The listing builds one solid part. Answer for the finished solid, in the listing's coordinates (mm). Face numbers are marked on the shaded views. Coordinates: 2 decimals unless noted, no trailing zeros. Loops run counter-clockwise (first coordinate to the right, second up) from the corner with the lowest first, then second, coordinate; pieces in that order, holes last. Notation, with made-up numbers: (-10.75, 58.5) - (8.25, 58.5) arc R32 ccw to (8.25, 97.5) - close; hole circle Ø11 at (9, 89.25). An arc over 180 degrees is marked (long way). Return JSON: item names as keys, results as strings. Group by question number.
1. Section C-C (z = 23) is taken. Write down the section's boundary in (x, y), and give its area (3 significant figures).
2. Each of these flat-tipped pins is pushed along its axis until it touches: P1, Ø3, axis at x = -8, y = -12, coming from the +Z side; P2, Ø3, axis at x = 7.5, y = -9.5, coming from the -Z side; P3, Ø2.5, axis at x = -13, y = -13, coming from the +Z side; P4, Ø4, axis at y = -3, z = 24.5, coming from the -X side. Where does it stop, or does it pass through?
3. Section B-B (x = -13) is taken. Write down the section's boundary in (y, z), and give its area (3 significant figures).
4. Section A-A (y = 0) is taken. Write down the section's boundary in (x, z).
5. Find the intervals of material crossed by line 1 along Y through (x, z) = (13, 15.95); line 2 along Z through (x, y) = (16, 2.5); line 3 along Z through (x, y) = (0.5, 7), in increasing order.
6. Section D-D (y = 4.5) is taken. Write down the section's boundary in (x, z).
7. The mould has two halves that part along Y. Classify the marked faces 1, 2 and 3: pulls with the +Y half, pulls with the -Y half, needs draft (parallel to the pull), parting line crosses it, or undercut.
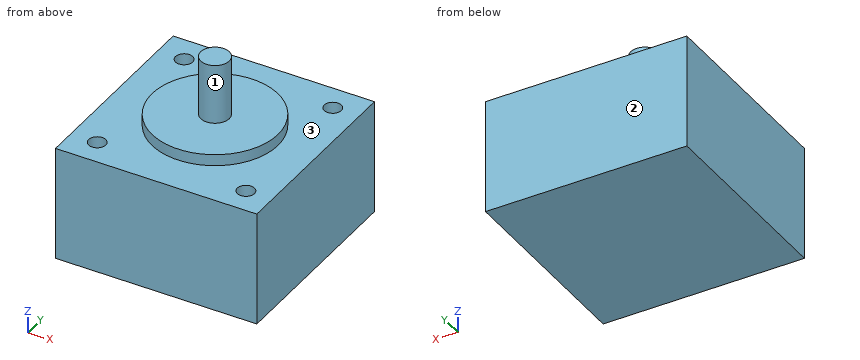
```python
from build123d import *

# Parameters (mm, degrees)
F0_W     = 35.2
F0_H     = 35.2
F1_DEPTH = 20
F2_R     = 11
F3_DEPTH = 2
F4_R     = 2.5
F5_DEPTH = 12.5
F6_R     = 1.5
F7_DEPTH = 6


with BuildPart() as f1:
    # F0 (on Top) → F1 (new body)
    with BuildSketch(Plane.XY):
        Rectangle(F0_W, F0_H)
    extrude(amount=F1_DEPTH)

    # F2 (on face) → F3 (join)
    with BuildSketch(Plane.XY.offset(20)):
        Circle(F2_R)
    extrude(amount=F3_DEPTH)

    # F4 (on face) → F5 (join)
    with BuildSketch(Plane.XY.offset(20)):
        Circle(F4_R)
    extrude(amount=F5_DEPTH)

    # F6 (on face) → F7 (cut)
    with BuildSketch(Plane.XY.offset(20)):
        with Locations((-13, 13)):
            Circle(F6_R)
        with Locations((13, 13)):
            Circle(F6_R)
        with Locations((-13, -13)):
            Circle(F6_R)
        with Locations((13, -13)):
            Circle(F6_R)
    extrude(amount=-F7_DEPTH, mode=Mode.SUBTRACT)


solid = f1.part
```
The answers:
{
 "1": {"outline": "circle Ø5 at (0, 0)", "area": "19.6 mm2"},
 "2": {"P1": "stops at z = 20", "P2": "stops at z = 0", "P3": "stops at z = 14", "P4": "stops at x = -2.29"},
 "3": {"outline": "(-17.6, 0) - (17.6, 0) - (17.6, 20) - (14.5, 20) - (14.5, 14) - (11.5, 14) - (11.5, 20) - (-11.5, 20) - (-11.5, 14) - (-14.5, 14) - (-14.5, 20) - (-17.6, 20) - close", "area": "668 mm2"},
 "4": {"outline": "(-17.6, 0) - (17.6, 0) - (17.6, 20) - (11, 20) - (11, 22) - (2.5, 22) - (2.5, 32.5) - (-2.5, 32.5) - (-2.5, 22) - (-11, 22) - (-11, 20) - (-17.6, 20) - close"},
 "5": {"line 1": "y = -17.6 to -14.5, -11.5 to 11.5, 14.5 to 17.6", "line 2": "z = 0 to 20", "line 3": "z = 0 to 22"},
 "6": {"outline": "(-17.6, 0) - (17.6, 0) - (17.6, 20) - (10.04, 20) - (10.04, 22) - (-10.04, 22) - (-10.04, 20) - (-17.6, 20) - close"},
 "7": {"face 1": "parting line crosses it", "face 2": "pulls with the +Y half", "face 3": "needs draft"}
}
